Check sheet for the modelled part. Datum: model origin and axes. Units: mm. Coordinates: 2 decimals unless noted, no trailing zeros. Loops run counter-clockwise (first coordinate to the right, second up) from the corner with the lowest first, then second, coordinate; pieces in that order, holes last. Notation, with made-up numbers: (86.25, -29.5) - (111.25, -29.5) arc R27 cw to (111.25, -3.5) - close; hole circle Ø6 at (21, 21). An arc over 180 degrees is marked (long way). Answer as a JSON object with one key per item and string values. Group by question number.
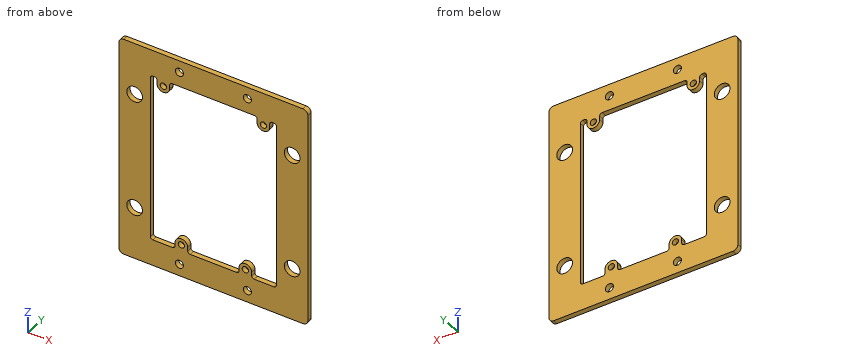
from build123d import *

# Parameters (mm, degrees)
SKETCH1_W           = 120
SKETCH1_H           = 142.16
BOSS_EXTRUDE1_DEPTH = 3.175
SKETCH2_R           = 5
CUT_EXTRUDE1_DEPTH  = 94.072267755
SKETCH3_R           = 2
CUT_EXTRUDE2_DEPTH  = 94.072267755
SKETCH4_R           = 2.5796875
CUT_EXTRUDE3_DEPTH  = 94.072267755
FILLET1_R           = 1.5875
FILLET2_R           = 3.175


with BuildPart() as part:
    # Sketch1 → Boss-Extrude1 (new body)
    with BuildSketch(Plane(origin=(0, 0, 0), x_dir=(1, 0, 0), z_dir=(0, 1, 0))):
        Rectangle(SKETCH1_W, SKETCH1_H)
    extrude(amount=BOSS_EXTRUDE1_DEPTH)

    # Sketch2 → Cut-Extrude1 (cut, through all)
    with BuildSketch(Plane(origin=(0, 3.175, 0), x_dir=(1, 0, 0), z_dir=(0, 1, 0))):
        with Locations(Location((-50, -37.5, 0), (0, 0, 270))):
            Circle(SKETCH2_R)
        with Locations(Location((50, -37.5, 0), (0, 0, 270))):
            Circle(SKETCH2_R)
        with Locations(Location((50, 37.5, 0), (0, 0, 270))):
            Circle(SKETCH2_R)
        with Locations(Location((-50, 37.5, 0), (0, 0, 270))):
            Circle(SKETCH2_R)
    extrude(amount=-CUT_EXTRUDE1_DEPTH, mode=Mode.SUBTRACT)

    # Sketch3 → Cut-Extrude2 (cut, through all)
    with BuildSketch(Plane(origin=(0, 3.175, 0), x_dir=(1, 0, 0), z_dir=(0, 1, 0))):
        with Locations(Location((31.75, -50.165011564, 0), (0, 0, 270))):
            Circle(SKETCH3_R)
        with Locations(Location((-31.75, -50.165011564, 0), (0, 0, 270))):
            Circle(SKETCH3_R)
        with Locations(Location((20.32, 50.165011564, 0), (0, 0, 270))):
            Circle(SKETCH3_R)
        with Locations(Location((-20.32, 50.165011564, 0), (0, 0, 270))):
            Circle(SKETCH3_R)
        with BuildLine():
            Line((-16.32, 50.165011564), (-16.32, 54.165011564))
            Line((-16.32, 54.165011564), (16.32, 54.165011564))
            Line((16.32, 54.165011564), (16.32, 50.165011564))
            ThreePointArc((16.32, 50.165011564), (20.32, 46.165011564), (24.32, 50.165011564))
            Line((24.32, 50.165011564), (24.32, 54.165011564))
            Line((24.32, 54.165011564), (40, 54.165011564))
            Line((40, 54.165011564), (40, -54.165011564))
            Line((40, -54.165011564), (35.75, -54.165011564))
            Line((35.75, -54.165011564), (35.75, -50.165011564))
            ThreePointArc((35.75, -50.165011564), (31.75, -46.165011564), (27.75, -50.165011564))
            Line((27.75, -50.165011564), (27.75, -54.165011564))
            Line((27.75, -54.165011564), (-27.75, -54.165011564))
            Line((-27.75, -54.165011564), (-27.75, -50.165011564))
            ThreePointArc((-27.75, -50.165011564), (-31.75, -46.165011564), (-35.75, -50.165011564))
            Line((-35.75, -50.165011564), (-35.75, -54.165011564))
            Line((-35.75, -54.165011564), (-40, -54.165011564))
            Line((-40, -54.165011564), (-40, 54.165011564))
            Line((-40, 54.165011564), (-24.32, 54.165011564))
            Line((-24.32, 54.165011564), (-24.32, 50.165011564))
            ThreePointArc((-24.32, 50.165011564), (-20.32, 46.165011564), (-16.32, 50.165011564))
        make_face()
    extrude(amount=-CUT_EXTRUDE2_DEPTH, mode=Mode.SUBTRACT)

    # Sketch4 → Cut-Extrude3 (cut, through all)
    with BuildSketch(Plane(origin=(0, 3.175, 0), x_dir=(1, 0, 0), z_dir=(0, 1, 0))):
        with Locations(Location((-21.59, 63.5, 0), (0, 0, 270))):
            Circle(SKETCH4_R)
        with Locations(Location((21.59, 63.5, 0), (0, 0, 270))):
            Circle(SKETCH4_R)
        with Locations(Location((-21.59, -63.5, 0), (0, 0, 90))):
            Circle(SKETCH4_R)
        with Locations(Location((21.59, -63.5, 0), (0, 0, 90))):
            Circle(SKETCH4_R)
    extrude(amount=-CUT_EXTRUDE3_DEPTH, mode=Mode.SUBTRACT)

    # Fillet1
    fillet1_edges = [part.edges().sort_by_distance(p)[0] for p in [
        (-16.32, 1.5875, -54.165011564),
        (16.32, 1.5875, -54.165011564),
        (24.32, 1.5875, -54.165011564),
        (40, 1.5875, -54.165011564),
        (40, 1.5875, 54.165011564),
        (35.75, 1.5875, 54.165011564),
        (27.75, 1.5875, 54.165011564),
        (-27.75, 1.5875, 54.165011564),
        (-35.75, 1.5875, 54.165011564),
        (-40, 1.5875, 54.165011564),
        (-40, 1.5875, -54.165011564),
        (-24.32, 1.5875, -54.165011564),
    ]]
    fillet(fillet1_edges, radius=FILLET1_R)

    # Fillet2
    fillet2_edges = [part.edges().sort_by_distance(p)[0] for p in [
        (60, 1.5875, 71.08),
        (-60, 1.5875, 71.08),
        (-60, 1.5875, -71.08),
        (60, 1.5875, -71.08),
    ]]
    fillet(fillet2_edges, radius=FILLET2_R)


solid = part.part
1. Sectioned sample at B-B on z = 63.5. Record the cut outline in (x, y) (3 decimals).
2. Gauge pin test, flat end, axial feed: pin 1 (11.5 mm diameter, centred on x = -50, z = -37.5, fed in from +Y) (3 decimals). Record the tip position at first contact, or that the pin passes through.
3. Sectioned sample at C-C on z = -3. Record the cut outline in (x, y) (3 decimals).
4. Sectioned sample at A-A on x = -31.75. Record the cut outline in (y, z) (3 decimals).
5. Material ranges on line 1 (Z direction, x = 31.5, y = 2.25); line 2 (X direction, y = 3.05, z = -50); line 3 (Z direction, x = -14, y = 0.6), recorded low to high.
6. Sectioned sample at D-D on z = 37.5. Record the cut outline in (x, y) (3 decimals), plus the area to 3 significant figures.
Answers follow:
{
 "1": {"outline": "(-60, 0) - (-24.17, 0) - (-24.17, 3.175) - (-60, 3.175) - close; (-19.01, 0) - (19.01, 0) - (19.01, 3.175) - (-19.01, 3.175) - close; (24.17, 0) - (60, 0) - (60, 3.175) - (24.17, 3.175) - close"},
 "2": {"pin 1": "stops at y = 3.175"},
 "3": {"outline": "(-60, 0) - (-40, 0) - (-40, 3.175) - (-60, 3.175) - close; (40, 0) - (60, 0) - (60, 3.175) - (40, 3.175) - close"},
 "4": {"outline": "(0, -71.08) - (3.175, -71.08) - (3.175, -54.165) - (0, -54.165) - close; (0, 46.165) - (3.175, 46.165) - (3.175, 48.165) - (0, 48.165) - close; (0, 52.165) - (3.175, 52.165) - (3.175, 71.08) - (0, 71.08) - close"},
 "5": {"line 1": "z = -71.08 to -54.17, 46.17 to 48.18, 52.15 to 71.08", "line 2": "x = -60 to -40, -24.32 to -22.31, -18.33 to -16.32, 16.32 to 18.33, 22.31 to 24.32, 40 to 60", "line 3": "z = -71.08 to -54.17, 54.17 to 71.08"},
 "6": {"outline": "(-60, 0) - (-55, 0) - (-55, 3.175) - (-60, 3.175) - close; (-45, 0) - (-40, 0) - (-40, 3.175) - (-45, 3.175) - close; (40, 0) - (45, 0) - (45, 3.175) - (40, 3.175) - close; (55, 0) - (60, 0) - (60, 3.175) - (55, 3.175) - close", "area": "63.5 mm^2"}
}
